Input: part model. Units: mm. Frame: model coordinates. Face numbers are marked on the shaded views. A direction names the side the tool comes from. Round coordinates to 2 decimals unless told otherwise and drop trailing zeros. Loops run counter-clockwise (first coordinate to the right, second up) from the corner with the lowest first, then second, coordinate; pieces in that order, holes last.
(1) Access query for the marked faces 1, 2 and 3. Directions: +Z, -Z, +X, -X, +Y, -Y. A direction counts if a zero-diameter tool reaches every point of the face in a straight line with its end or side. Return the directions, or none.
(2) Draft query along X for the marked faces 4, 5 and 6. Return one class per face: released by +X, released by -X, zero draft, split by the parting line, or undercut.
(3) Cut plane D-D, the plane x = 23. Output: boundary loops of the cut face in (y, z), and give its area (3 significant figures).
(4) First-contact query: pin 1 Ø7.5 at (x, z) = (-10, 22.5) entering from +Y; pin 2 Ø1.5 at (x, z) = (13.5, 39.5) entering from +Y; pin 3 Ø16 at (x, y) = (-7.5, -22.59) entering from +Z; pin 4 Ø4 at (x, z) = (-6.5, 29) entering from -Y. Flat tips, straight axial feed; report the tip coordinate or a pass-through.
(5) Cut plane B-B, the plane x = -10. Output: boundary loops of the cut face in (y, z), and give its area (3 significant figures).
(6) Cut plane A-A, the plane z = 18. Output: boundary loops of the cut face in (x, y), and give its area (3 significant figures).
(7) Cut plane C-C, the plane y = -24.5. Output: boundary loops of the cut face in (x, z).
(8) Line query: line 1 (X direction, y = -26, z = 20); line 2 (Y direction, x = 13.5, z = 11.5); line 3 (X direction, y = -28.5, z = 19.5). Output: solid intervals per line, ascending.
from build123d import *

# Parameters (mm, degrees)
ESQUISSE1_R        = 7
BOSS_EXTRU_2_DEPTH = 45


with BuildPart() as part:
    # Esquisse1 → Boss.-Extru.2 (new body)
    with BuildSketch(Plane.XY):
        with BuildLine():
            Line((33.502581987, 1.407665382), (57.502581987, 1.407665382))
            Line((57.502581987, 1.407665382), (62.502581987, -3.592334618))
            Line((62.502581987, -3.592334618), (62.502581987, -22.592334618))
            Line((62.502581987, -22.592334618), (33.502581987, -57.592334618))
            Line((33.502581987, -57.592334618), (29.502581987, -57.592334618))
            ThreePointArc((29.502581987, -57.592334618), (24.333450387, -50.001682761), (21.96277386, -41.129376977))
            ThreePointArc((21.96277386, -41.129376977), (20.352131518, -37.896743447), (16.984252973, -36.592334618))
            Line((16.984252973, -36.592334618), (-14.497418013, -36.592334618))
            Line((-14.497418013, -36.592334618), (-21.497418013, -29.592334618))
            Line((-21.497418013, -29.592334618), (-21.497418013, -11.592334618))
            Line((-21.497418013, -11.592334618), (-14.497418013, -4.592334618))
            Line((-14.497418013, -4.592334618), (-7.497418013, -4.592334618))
            Line((-7.497418013, -4.592334618), (13.477054889, -8.290700097))
            ThreePointArc((13.477054889, -8.290700097), (25.057973951, -6.679500169), (33.502581987, 1.407665382))
        make_face()
        with Locations(Location((-7.497418013, -22.592334618, 0), (0, 0, 180))):
            Circle(ESQUISSE1_R, mode=Mode.SUBTRACT)
    extrude(amount=BOSS_EXTRU_2_DEPTH)


solid = part.part
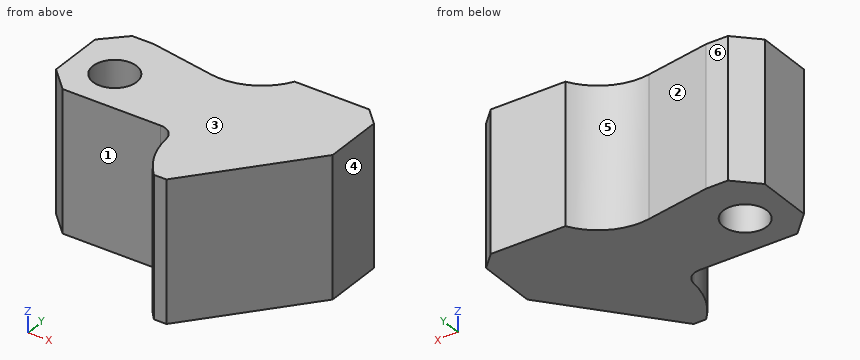
Reported:
1. face 1: +Z, -Z, -X, -Y
1. face 2: +Z, -Z, +Y
1. face 3: +Z, +X, -X, +Y, -Y
2. face 4: released by +X
2. face 5: undercut
2. face 6: zero draft
3. outline: (-46.46, 0) - (-7.53, 0) - (-7.53, 45) - (-46.46, 45) - close
3. area: 1,750 mm2
4. pin 1: stops at y = -4.59
4. pin 2: stops at y = -8.16
4. pin 3: stops at z = 45
4. pin 4: stops at y = -36.59
5. outline: (-36.59, 0) - (-29.13, 0) - (-29.13, 45) - (-36.59, 45) - close; (-16.05, 0) - (-4.59, 0) - (-4.59, 45) - (-16.05, 45) - close
5. area: 852 mm2
6. outline: (-21.5, -29.59) - (-14.5, -36.59) - (16.98, -36.59) arc R5 cw to (21.96, -41.13) arc R27.4 ccw to (29.5, -57.59) - (33.5, -57.59) - (62.5, -22.59) - (62.5, -3.59) - (57.5, 1.41) - (33.5, 1.41) arc R19 cw to (13.48, -8.29) - (-7.5, -4.59) - (-14.5, -4.59) - (-21.5, -11.59) - close; hole circle Ø14 at (-7.5, -22.59)
6. area: 2,880 mm2
7. outline: (-21.5, 0) - (-14.23, 0) - (-14.23, 45) - (-21.5, 45) - close; (-0.76, 0) - (60.92, 0) - (60.92, 45) - (-0.76, 45) - close
8. line 1: x = -21.5 to -13.61, -1.38 to 59.68
8. line 2: y = -36.59 to -8.29
8. line 3: x = -21.5 to -11.25, -3.74 to 57.61
